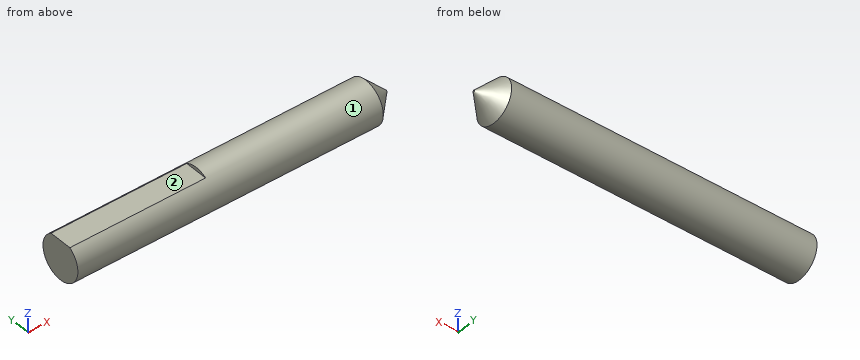
```python
from build123d import *

# Parameters (mm, degrees)
F0_W     = 48
F0_H     = 3.15
F2_SIZE  = 3
F4_DEPTH = 20


with BuildPart() as f1:
    # F0 (on Front) → F1 (revolve)
    with BuildSketch(Plane.XZ):
        with Locations((24, 1.575)):
            Rectangle(F0_W, F0_H)
    revolve(axis=Axis((24, 0, 0), (-1, 0, 0)))

    # F2
    f2_edges = [f1.edges().sort_by_distance(p)[0] for p in [
        (48, 0, -3.15),
    ]]
    chamfer(f2_edges, length=F2_SIZE)

    # F3 (on face) → F4 (cut)
    with BuildSketch(Plane(origin=(0, 0, 0), x_dir=(0, -1, 0), z_dir=(-1, 0, 0))):
        with BuildLine():
            Line((-1.7029386366, 2.65), (1.7029386366, 2.65))
            ThreePointArc((1.7029386366, 2.65), (0.8874119675, 3.0224162519), (0, 3.15))
            ThreePointArc((0, 3.15), (-0.8874119675, 3.0224162519), (-1.7029386366, 2.65))
        make_face()
    extrude(amount=-F4_DEPTH, mode=Mode.SUBTRACT)


solid = f1.part
```
Here's how the part is built. I have some questions about the finished solid (model axes, mm). Face numbers are marked on the shaded views. A direction names the side the tool comes from. Coordinates: 2 decimals unless noted, no trailing zeros. Order: outer loops, then holes, each group sorted by start corner. A loop starts at its lowest first (then second) coordinate and runs counter-clockwise, first axis right, second up. Notation, with made-up numbers: (-26, 36) -> (20, 36) arc R22 ccw to (20, 46) -> close; hole circle Ø11 at (-17.75, 34.5). An arc over 180 degrees is marked (long way). Return JSON: item names as keys, results as strings.
1) If we section it at A-A on x = 43.5: List the corners of the cut face in (y, z) for me.
Conclusion:
{"outline": "circle Ø6.3 at (0, 0)"}
2) On a 3-axis mill with a long thin cutter (end or side, diameter ignored), from which of +Z, -Z, +X, -X, +Y, -Y can I reach the whole of each face in a straight line? I mean the marked faces 1 and 2. Say none if no direction works.
Conclusion:
{"face 1": "+X, -X", "face 2": "+Z, -X, +Y, -Y"}
3) If I drill on probe 1 along Z at (x, y) = (2, -1); probe 2 along Y at (x, z) = (10.5, 1.75); probe 3 along X at (y, z) = (-0.75, 0.75), over which ranges is the centre line in solid material (lowest first)?
Conclusion:
{"probe 1": "z = -2.99 to 2.65", "probe 2": "y = -2.62 to 2.62", "probe 3": "x = 0 to 47.09"}
4) I'm going to push flat-ended pins straight in: P1, Ø1.5, axis at x = 12, z = -2, coming from the +Y side; P2, Ø1, axis at x = 12.5, y = -0.5, coming from the +Z side; P3, Ø3, axis at x = 10, y = 2, coming from the -Z side. Where does each tip first touch, or does it pass through?
Conclusion:
{"P1": "stops at y = 2.89", "P2": "stops at z = 2.65", "P3": "stops at z = -3.11"}
